from build123d import *

# Parameters (mm, degrees)
SKETCH1_R                          = 193.675
BOSS_EXTRUDE1_DEPTH                = 6.35
F_9_0_196_DIAMETER_HOLE1_D         = 4.9784
SKETCH5_R                          = 82.55
CUT_EXTRUDE1_DEPTH                 = 6.35
F_9_0_196_DIAMETER_HOLE2_D         = 4.9784
F_9_0_196_DIAMETER_HOLE3_OUTLINE_R = 2.4892
F_9_0_196_DIAMETER_HOLE3_DEPTH     = 6.35


# Read off the part's stored shape, not the designer's step: #9 (0.196) Diameter Hole3
with BuildPart() as part:
    # Sketch1 → Boss-Extrude1 (new body)
    with BuildSketch(Plane(origin=(0, 0, 0), x_dir=(0, 1, 0), z_dir=(0, 0, 1))):
        with Locations(Location((0, 0, 0), (0, 0, 270))):
            Circle(SKETCH1_R)
    extrude(amount=BOSS_EXTRUDE1_DEPTH)

    # #9 (0.196) Diameter Hole1 (through all)
    with Locations(Plane.XY.offset(6.35)):
        with Locations((-150.657762959, 86.9823), (-173.9646, 0), (-150.657762959, -86.9823), (-86.9823, -150.657762959), (0, -173.9646), (86.9823, -150.657762959), (150.657762959, -86.9823), (173.9646, 0), (150.657762959, 86.9823), (86.9823, 150.657762959), (0, 173.9646), (-86.9823, 150.657762959)):
            Hole(F_9_0_196_DIAMETER_HOLE1_D / 2)

    # Sketch5 → Cut-Extrude1 (cut)
    with BuildSketch(Plane.XY.offset(6.35)):
        Circle(SKETCH5_R)
    extrude(amount=-CUT_EXTRUDE1_DEPTH, mode=Mode.SUBTRACT)

    # #9 (0.196) Diameter Hole2 (through all)
    with Locations(Plane.XY.offset(6.35)):
        with Locations((101.6, 92.075), (101.6, 79.375), (101.6, 66.675), (101.6, 53.975), (101.6, 41.275), (101.6, 28.575), (101.6, 15.875), (101.6, 3.175), (101.6, -9.525), (101.6, -22.225), (101.6, -34.925), (-101.6, 92.075), (-101.6, 79.375), (-101.6, 66.675), (-101.6, 53.975), (-101.6, 41.275), (-101.6, 28.575), (-101.6, 15.875), (-101.6, 3.175), (-101.6, -9.525), (-101.6, -22.225), (-101.6, -34.925)):
            Hole(F_9_0_196_DIAMETER_HOLE2_D / 2)

    # #9 (0.196) Diameter Hole3 outline → #9 (0.196) Diameter Hole3 (cut)
    with BuildSketch(Plane.XY):
        with Locations((66.250745249, -91.186327978)):
            Circle(F_9_0_196_DIAMETER_HOLE3_OUTLINE_R)
        with Locations((58.785872545, -80.91181215)):
            Circle(F_9_0_196_DIAMETER_HOLE3_OUTLINE_R)
        with Locations((107.195957593, -34.830077978)):
            Circle(F_9_0_196_DIAMETER_HOLE3_OUTLINE_R)
        with Locations((95.117539836, -30.90556215)):
            Circle(F_9_0_196_DIAMETER_HOLE3_OUTLINE_R)
        with Locations((107.195957593, 34.830077978)):
            Circle(F_9_0_196_DIAMETER_HOLE3_OUTLINE_R)
        with Locations((95.117539836, 30.90556215)):
            Circle(F_9_0_196_DIAMETER_HOLE3_OUTLINE_R)
        with Locations((66.250745249, 91.186327978)):
            Circle(F_9_0_196_DIAMETER_HOLE3_OUTLINE_R)
        with Locations((58.785872545, 80.91181215)):
            Circle(F_9_0_196_DIAMETER_HOLE3_OUTLINE_R)
        with Locations((0, 112.7125)):
            Circle(F_9_0_196_DIAMETER_HOLE3_OUTLINE_R)
        with Locations((0, 100.0125)):
            Circle(F_9_0_196_DIAMETER_HOLE3_OUTLINE_R)
        with Locations((-66.250745249, 91.186327978)):
            Circle(F_9_0_196_DIAMETER_HOLE3_OUTLINE_R)
        with Locations((-58.785872545, 80.91181215)):
            Circle(F_9_0_196_DIAMETER_HOLE3_OUTLINE_R)
        with Locations((-107.195957593, 34.830077978)):
            Circle(F_9_0_196_DIAMETER_HOLE3_OUTLINE_R)
        with Locations((-95.117539836, 30.90556215)):
            Circle(F_9_0_196_DIAMETER_HOLE3_OUTLINE_R)
        with Locations((-107.195957593, -34.830077978)):
            Circle(F_9_0_196_DIAMETER_HOLE3_OUTLINE_R)
        with Locations((-95.117539836, -30.90556215)):
            Circle(F_9_0_196_DIAMETER_HOLE3_OUTLINE_R)
        with Locations((-66.250745249, -91.186327978)):
            Circle(F_9_0_196_DIAMETER_HOLE3_OUTLINE_R)
        with Locations((-58.785872545, -80.91181215)):
            Circle(F_9_0_196_DIAMETER_HOLE3_OUTLINE_R)
        with Locations((0, -112.7125)):
            Circle(F_9_0_196_DIAMETER_HOLE3_OUTLINE_R)
        with Locations((0, -100.0125)):
            Circle(F_9_0_196_DIAMETER_HOLE3_OUTLINE_R)
    extrude(amount=F_9_0_196_DIAMETER_HOLE3_DEPTH, mode=Mode.SUBTRACT)


solid = part.part
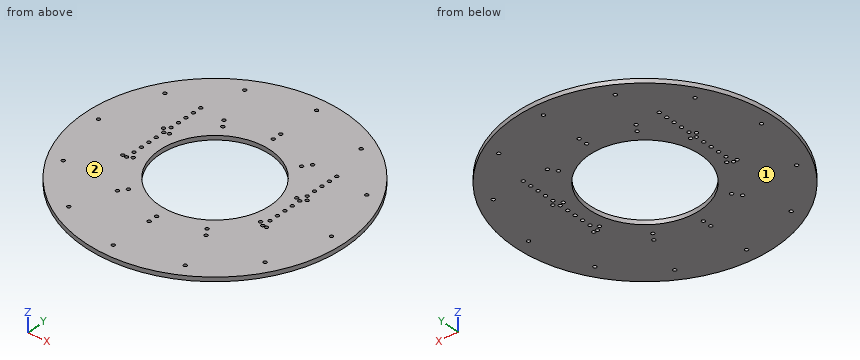
Geometry: final body of the model. Coordinates: model frame, mm. Face numbers are marked on the shaded views. Coordinates: 2 decimals unless noted, no trailing zeros. Order: outer loops, then holes, each group sorted by start corner. A loop starts at its lowest first (then second) coordinate and runs counter-clockwise, first axis right, second up.
1) Section A-A (x = 33.5). Return loops of the section in (y, z), then the cut area to 3 significant figures.
Result sheet:
outline: (-190.76, 0) - (-75.45, 0) - (-75.45, 6.35) - (-190.76, 6.35) - close; (75.45, 0) - (190.76, 0) - (190.76, 6.35) - (75.45, 6.35) - close
area: 1,460 mm2
2) First-contact query: P1, Ø4.5, axis at x = 86.98, y = 150.66, coming from the +Z side; P2, Ø1.5, axis at y = 101, z = 4, coming from the -X side; P3, Ø1, axis at y = -70, z = 4.5, coming from the +X side; P4, Ø1, axis at x = 58, z = 4.5, coming from the -Y side. Flat tips, straight axial feed; report the tip coordinate or a pass-through.
Result sheet:
P1: passes through
P2: stops at x = -165.71
P3: stops at x = 180.78
P4: stops at y = -184.94
3) Section B-B (z = 2.5). Give the number of separate pieces and of enclosed holes in the cut face, then the cut area to 3 significant figures.
Result sheet:
separate pieces: 1
enclosed holes: 55
area: 95,400 mm2
4) Ray query, probe 1 along Y at (x, z) = (97, 3.5); probe 2 along X at (y, z) = (-151.5, 5); probe 3 along Y at (x, z) = (93, 5). Return the intervals inside material, ascending.
Result sheet:
probe 1: y = -167.63 to -32.53, -29.28 to 29.28, 32.53 to 167.63
probe 2: x = -120.66 to -89.32, -84.64 to 84.64, 89.32 to 120.66
probe 3: y = -169.89 to -32.21, -29.6 to 29.6, 32.21 to 169.89
5) Draft query along Z for the marked faces 1 and 2. Return one class per face: released by +Z, released by -Z, zero draft, split by the parting line, or undercut.
Result sheet:
face 1: released by -Z
face 2: released by +Z
6) Section C-C (y = -127.5). Return loops of the section in (x, z).
Result sheet:
outline: (-145.79, 0) - (145.79, 0) - (145.79, 6.35) - (-145.79, 6.35) - close
